from build123d import *

# Parameters (mm, degrees)
SKETCH1_R           = 3
SKETCH1_R_2         = 1.6
BOSS_EXTRUDE1_DEPTH = 3
SKETCH2_R           = 1.3
CUT_EXTRUDE1_DEPTH  = 3
BOSS_EXTRUDE2_START = -3
BOSS_EXTRUDE2_DEPTH = 3


with BuildPart() as part:
    # Sketch1 → Boss-Extrude1 (new body)
    with BuildSketch(Plane(origin=(0, 0, 0), x_dir=(1, 0, 0), z_dir=(0, 1, 0))):
        with BuildLine():
            Line((-4.531642246, 17.7995776), (-7.838367177, 1.6))
            ThreePointArc((-7.838367177, 1.6), (0, -8), (7.838367177, 1.6))
            Line((7.838367177, 1.6), (4.531642246, 17.7995776))
            ThreePointArc((4.531642246, 17.7995776), (0, 21.499648), (-4.531642246, 17.7995776))
        make_face()
        with Locations(Location((0, 16.87456, 0), (0, 0, 270))):
            Circle(SKETCH1_R, mode=Mode.SUBTRACT)
        with Locations(Location((0, 0, 0), (0, 0, 270))):
            Circle(SKETCH1_R_2, mode=Mode.SUBTRACT)
    extrude(amount=BOSS_EXTRUDE1_DEPTH)

    # Sketch2 → Cut-Extrude1 (cut)
    with BuildSketch(Plane(origin=(0, 3, 0), x_dir=(1, 0, 0), z_dir=(0, 1, 0))):
        with Locations(Location((0, 6.35, 0), (0, 0, 270))):
            Circle(SKETCH2_R)
        with Locations(Location((6.35, 0, 0), (0, 0, 270))):
            Circle(SKETCH2_R)
        with Locations(Location((0, -6.35, 0), (0, 0, 270))):
            Circle(SKETCH2_R)
        with Locations(Location((-6.35, 0, 0), (0, 0, 270))):
            Circle(SKETCH2_R)
    extrude(amount=-CUT_EXTRUDE1_DEPTH, mode=Mode.SUBTRACT)

    # Sketch3 → Boss-Extrude2 (add)
    with BuildSketch(Plane(origin=(0, 3, 0), x_dir=(1, 0, 0), z_dir=(0, 1, 0)).offset(BOSS_EXTRUDE2_START)):
        with BuildLine():
            Line((-7.838367177, 1.6), (-6.8136721, 6.619960159))
            ThreePointArc((-6.8136721, 6.619960159), (0, -9.5), (6.8136721, 6.619960159))
            Line((6.8136721, 6.619960159), (7.838367177, 1.6))
            ThreePointArc((7.838367177, 1.6), (0, -8), (-7.838367177, 1.6))
        make_face()
    extrude(amount=BOSS_EXTRUDE2_DEPTH)


solid = part.part
Part model, mm, in its own coordinate system. Give positions to 0.01 mm unless a question says otherwise; leave off trailing zeros. Loops run counter-clockwise (first coordinate to the right, second up) from the corner with the lowest first, then second, coordinate; pieces in that order, holes last. Notation, with made-up numbers: M 12.25,-3 L 21.25,-3 A21 cw 21.25,29 Z; hole C 32.25,62.5 d1. An arc over 180 degrees is marked long. Put each result on its own line as item: value. Start each with the question number.
1) Probe probe 1 along X at (y, z) = (2.25, 0); probe 2 along Z at (x, y) = (-0.25, 1.45) (3 decimals); probe 3 along X at (y, z) = (2.5, 7.5). List the from-to ranges inside material, lowest first.
2) Saw through at C-C (z = 0). List the corners of the cut face in (x, y).
3) Saw through at A-A (x = 0). List the corners of the cut face in (y, z).
4) Pull direction X, two halves, no side cores. Call faces 1 (the cylindrical face through (-0.311, 1.479, 9.495)), 2 (the flat face through (5.69, 1.48, -12.13)), 3 (the flat face through (0, 0, -3)), 4 (the cylindrical face through (0.06, 1.52, 5.05)): +X half, -X half, draft (parallel to the pull), parting line (faces both ways), or undercut.
5) Saw through at D-D (z = 6.35). List the corners of the cut face in (x, y).
6) Saw through at B-B (y = 1.05). List the corners of the cut face in (x, z).
7) Flat gauge pin, fed straight in: pin 1 (8 mm diameter, centred on x = 0, z = -16.87, fed in from -Y). Where does the tip first touch, or does it go through?
Numbers:
1. probe 1: -9.5 to -7.65, -5.05 to -1.6, 1.6 to 5.05, 7.65 to 9.5
1. probe 2: -21.493 to -19.864, -13.885 to -7.626, -5.074 to -1.58, 1.58 to 5.074, 7.626 to 9.497
1. probe 3: -5.83 to -0.61, 0.61 to 5.83
2. outline: M -9.5,0 L -7.65,0 L -7.65,3 L -9.5,3 Z; M -5.05,0 L -1.6,0 L -1.6,3 L -5.05,3 Z; M 1.6,0 L 5.05,0 L 5.05,3 L 1.6,3 Z; M 7.65,0 L 9.5,0 L 9.5,3 L 7.65,3 Z
3. outline: M 0,-21.5 L 3,-21.5 L 3,-19.87 L 0,-19.87 Z; M 0,-13.87 L 3,-13.87 L 3,-7.65 L 0,-7.65 Z; M 0,-5.05 L 3,-5.05 L 3,-1.6 L 0,-1.6 Z; M 0,1.6 L 3,1.6 L 3,5.05 L 0,5.05 Z; M 0,7.65 L 3,7.65 L 3,9.5 L 0,9.5 Z
4. face 1: parting line
4. face 2: +X half
4. face 3: draft
4. face 4: undercut
5. outline: M -7.07,0 L -1.3,0 L -1.3,3 L -7.07,3 Z; M 1.3,0 L 7.07,0 L 7.07,3 L 1.3,3 Z
6. outline: M -6.81,-6.62 L -4.53,-17.8 A4.63 ccw 4.53,-17.8 L 6.81,-6.62 A9.5 ccw long Z; hole C -6.35,0 d2.6; hole C 0,-16.87 d6; hole C 0,0 d3.2; hole C 0,-6.35 d2.6; hole C 0,6.35 d2.6; hole C 6.35,0 d2.6
7. pin 1: y = 0
